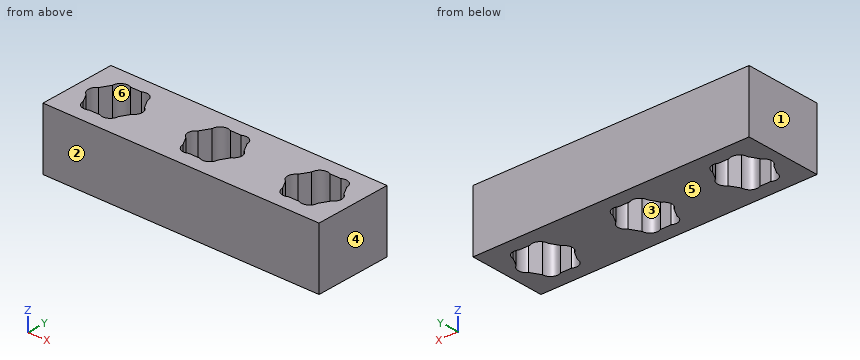
Autodesk Inventor part; units mm, degrees
ref_plane "YZ Plane" through (0, 0, 0) normal (1, 0, 0) x (0, 1, 0)
ref_plane "XZ Plane" through (0, 0, 0) normal (0, 1, 0) x (-1, 0, 0)
ref_plane "XY Plane" through (0, 0, 0) normal (0, 0, 1) x (1, 0, 0)
sketch "スケッチ1" plane through (0, 0, 0) normal (0, 0, 1) x (1, 0, 0)
  line L0 (-18, -5) -> (18, -5)
  line L1 (18, -5) -> (18, 5)
  line L2 (18, 5) -> (-18, 5)
  line L3 (-18, 5) -> (-18, -5)
  line L4 (-18, -5) -> (18, 5) construction
  line L5 (18, -5) -> (-18, 5) construction
  circle A0 centre (-13, 0) radius 1.55
  circle A1 centre (0, 0) radius 1.55
  line L6 (0, 0) -> (0, 5) construction
  line L7 (-12.5995, 5) -> (4.4005, 5) construction
  line L8 (-8.5, -4) -> (8.5, -4) construction
  line L9 (-11.2391, -3.05) -> (-14.7609, -3.05)
  line L10 (-14.7609, -3.05) -> (-16.5218, 0)
  line L11 (-16.5218, 0) -> (-14.7609, 3.05)
  line L12 (-14.7609, 3.05) -> (-11.2391, 3.05)
  line L13 (-11.2391, 3.05) -> (-9.4782, 0)
  line L14 (-9.4782, 0) -> (-11.2391, -3.05)
  circle A2 centre (-15.4718, 0) radius 1.05
  circle A3 centre (-14.2359, -2.1407) radius 1.05
  circle A4 centre (-11.7641, -2.1407) radius 1.05
  circle A5 centre (-10.5282, 0) radius 1.05
  circle A6 centre (-11.7641, 2.1407) radius 1.05
  circle A7 centre (-14.2359, 2.1407) radius 1.05
  circle A8 centre (13, 0) radius 1.55
  line L15 (11.2391, -3.05) -> (14.7609, -3.05)
  line L16 (14.7609, -3.05) -> (16.5218, 0)
  line L17 (16.5218, 0) -> (14.7609, 3.05)
  line L18 (14.7609, 3.05) -> (11.2391, 3.05)
  line L19 (11.2391, 3.05) -> (9.4782, 0)
  line L20 (9.4782, 0) -> (11.2391, -3.05)
  circle A9 centre (15.4718, 0) radius 1.05
  circle A10 centre (14.2359, -2.1407) radius 1.05
  circle A11 centre (11.7641, -2.1407) radius 1.05
  circle A12 centre (10.5282, 0) radius 1.05
  circle A13 centre (11.7641, 2.1407) radius 1.05
  circle A14 centre (14.2359, 2.1407) radius 1.05
  circle A15 centre (-13, 0) radius 5 construction
  line L21 (1.7609, -3.05) -> (-1.7609, -3.05)
  line L22 (-1.7609, -3.05) -> (-3.5218, 0)
  line L23 (-3.5218, 0) -> (-1.7609, 3.05)
  line L24 (-1.7609, 3.05) -> (1.7609, 3.05)
  line L25 (1.7609, 3.05) -> (3.5218, 0)
  line L26 (3.5218, 0) -> (1.7609, -3.05)
  circle A16 centre (-2.4718, 0) radius 1.05
  circle A17 centre (-1.2359, -2.1407) radius 1.05
  circle A18 centre (1.2359, -2.1407) radius 1.05
  circle A19 centre (2.4718, 0) radius 1.05
  circle A20 centre (1.2359, 2.1407) radius 1.05
  circle A21 centre (-1.2359, 2.1407) radius 1.05
  point P0 (-11.2391, -3.05)
  point P1 (-9.4782, 0)
  point P2 (-11.2391, 3.05)
  point P3 (-14.7609, 3.05)
  point P4 (11.2391, -3.05)
  point P5 (9.4782, 0)
  point P6 (11.2391, 3.05)
  point P7 (14.7609, 3.05)
  point P8 (-1.7609, -3.05)
  point P9 (1.7609, -3.05)
  point P10 (3.5218, 0)
  point P11 (1.7609, 3.05)
  point P12 (-1.7609, 3.05)
  dimension "d19" = 2.1
  dimension "d1" = 3.1
  dimension "d4" = 13
  dimension "d5" = 10
  dimension "d20" = 6.1
  dimension "d23" = 360
  dimension "d33" = 360
extrude "押し出し1" add sketch "スケッチ1" along normal blind 8
properties part number "胴体_サブフレーム_1_2" material "アセタール樹脂、黒"
Could you check a few things on this model? Use its own coordinates, in mm. Face numbers are marked on the shaded views. A direction names the side the tool comes from. Round coordinates to 2 decimals unless told otherwise and drop trailing zeros. Loops run counter-clockwise (first coordinate to the right, second up) from the corner with the lowest first, then second, coordinate; pieces in that order, holes last. Notation, with made-up numbers: M 60,-24.75 L 80,-24.75 A17 cw 80,-6.75 Z; hole C 58,49.5 d3. An arc over 180 degrees is marked long. Put each result on its own line as item: value.
Q1. Imagine slicing it at A-A (x = -1.5). Write out the boundary of the cut face in (y, z), then the cut area to 3 significant figures.
Check result:
outline: M -5,0 L -3.16,0 L -3.16,8 L -5,8 Z; M 3.16,0 L 5,0 L 5,8 L 3.16,8 Z
area: 29.5 mm2
Q2. Thinking about a two-plate mould opening in X: for the marked faces 1, 2, 3 and 4, which applies, released by +X, released by -X, zero draft, split by the parting line, or undercut?
Check result:
face 1: released by -X
face 2: zero draft
face 3: undercut
face 4: released by +X
Q3. I need wall thicknesses on probe 1 along X at (y, z) = (-2.25, 1); probe 2 along X at (y, z) = (1, 3); probe 3 along Y at (x, z) = (10, 1). Which ranges of each line are inside material? Lowest first, please.
Check result:
probe 1: -18 to -15.28, -10.72 to -2.28, 2.28 to 10.72, 15.28 to 18
probe 2: -18 to -15.94, -10.06 to -2.94, 2.94 to 10.06, 15.94 to 18
probe 3: -5 to -0.91, 0.91 to 5
Q4. Imagine slicing it at C-C (z = 1). State how many separate pieces and enclosed holes the cut face has, then the cut area to 3 significant figures.
Check result:
separate pieces: 1
enclosed holes: 3
area: 260 mm2
Q5. Imagine slicing it at B-B (y = 1.5). Write out the boundary of the cut face in (x, z), then the cut area to 3 significant figures.
Check result:
outline: M -18,0 L -15.66,0 L -15.66,8 L -18,8 Z; M -10.34,0 L -2.66,0 L -2.66,8 L -10.34,8 Z; M 2.66,0 L 10.34,0 L 10.34,8 L 2.66,8 Z; M 15.66,0 L 18,0 L 18,8 L 15.66,8 Z
area: 161 mm2
Q6. On a 3-axis mill with a long thin cutter (end or side, diameter ignored), from which of +Z, -Z, +X, -X, +Y, -Y can I reach the whole of each face in a straight line? I mean the marked faces 5 and 6. Say none if no direction works.
Check result:
face 5: -Z, +X, -X, +Y, -Y
face 6: +Z, -Z
